For this review, take the finished solid that the model builds, in its own axes (mm). A direction names the side the tool comes from. Give positions to 0.01 mm unless a question says otherwise; leave off trailing zeros. Loops run counter-clockwise (first coordinate to the right, second up) from the corner with the lowest first, then second, coordinate; pieces in that order, holes last. Notation, with made-up numbers: (25, -29.5) - (60, -29.5) arc R18 cw to (60, -0.5) - close; hole circle Ø10 at (72, 72.5). An arc over 180 degrees is marked (long way). Answer in a Markdown table with one row per item.
Autodesk Inventor part; units mm, degrees
ref_plane "YZ Plane" through (0, 0, 0) normal (1, 0, 0) x (0, 1, 0)
ref_plane "XZ Plane" through (0, 0, 0) normal (0, 1, 0) x (-1, 0, 0)
ref_plane "XY Plane" through (0, 0, 0) normal (0, 0, 1) x (1, 0, 0)
sketch "Sketch3" plane through (0, 0, 0) normal (0, 0, 1) x (1, 0, 0)
  line L0 (225, 240) -> (-225, 240)
  line L1 (-225, 240) -> (-225, -240)
  line L2 (-225, -240) -> (225, -240)
  line L3 (225, -240) -> (225, 240)
  line L4 (225, 240) -> (-225, -240) construction
  line L5 (-225, 240) -> (225, -240) construction
  line L6 (150, 180) -> (-150, 180)
  line L7 (-150, 180) -> (-150, -180)
  line L8 (-150, -180) -> (150, -180)
  line L9 (150, -180) -> (150, 180)
  line L10 (150, 180) -> (-150, -180) construction
  line L11 (-150, 180) -> (150, -180) construction
  point P0 (0, 0)
  dimension "d22" = 450
  dimension "d23" = 480
  dimension "d24" = 300
  dimension "d25" = 360
extrude "Plate3" add sketch "Sketch3" along normal blind 10
sketch "Sketch4" plane through (0, 0, 0) normal (0, 0, -1) x (-1, 0, 0)
  circle A0 centre (0, 230) radius 6.5
  circle A1 centre (195, 230) radius 6.5
  circle A2 centre (-195, 230) radius 6.5
  circle A3 centre (-200, 160) radius 6.5
  circle A4 centre (-200, 0) radius 6
  circle A5 centre (-200, -160) radius 6
  circle A6 centre (-195, -230) radius 6
  circle A7 centre (0, -230) radius 6
  circle A8 centre (195, -230) radius 6
  circle A9 centre (200, -160) radius 6.5
  circle A10 centre (200, 0) radius 6.5
  circle A11 centre (200, 160) radius 6.5
  point P0 (0, 0)
extrude "Cut1" cut sketch "Sketch4" against normal blind 10
equation "\"d26\" = Thickness"
equation "\"d18\" = Thickness"
equation "\"BendReliefDepth\" = 0.5 * Thickness"
properties part number "NVPH-305 main flange"
1. For faces 4 (the face through (150, -3, 5)), 5 (the face through (3, 240, 5)), list the 3-axis set-ups (+Z, -Z, +X, -X, +Y, -Y) from which the entire face can be reached by the end or side of a thin tool; tool diameter is ignored.
Values:
| item | result |
|---|---|
| face 4 | +Z, -Z |
| face 5 | +Z, -Z, +X, -X, +Y |
2. We need section A-A, the plane y = 230. Give the boundary of the cut face in (x, z).
Values:
| item | result |
|---|---|
| outline | (-225, 0) - (-201.5, 0) - (-201.5, 10) - (-225, 10) - close; (-188.5, 0) - (-6.5, 0) - (-6.5, 10) - (-188.5, 10) - close; (6.5, 0) - (188.5, 0) - (188.5, 10) - (6.5, 10) - close; (201.5, 0) - (225, 0) - (225, 10) - (201.5, 10) - close |
3. Clearance check with a flat-ended pin moving along its axis: pin 1 (15 mm diameter, centred on x = 200, y = 160, fed in from -Z). State where the tip first meets the part, or that it passes through.
Values:
| item | result |
|---|---|
| pin 1 | stops at z = 0 |
4. Wall thickness on line 1 (Y direction, x = 132, z = 3); line 2 (X direction, y = -135, z = 2); line 3 (Y direction, x = -199.5, z = 2.75): over which ranges is each line inside the solid? List them lowest first. Write a range as [from, to].
Values:
| item | result |
|---|---|
| line 1 | y = [-240, -180], [180, 240] |
| line 2 | x = [-225, -150], [150, 225] |
| line 3 | y = [-240, -233.97], [-226.03, -166.48], [-153.52, -6.48], [6.48, 153.52], [166.48, 225.31], [234.69, 240] |
5. We need section D-D, the plane y = -84. Give the boundary of the cut face in (x, z), and give its area (3 significant figures).
Values:
| item | result |
|---|---|
| outline | (-225, 0) - (-150, 0) - (-150, 10) - (-225, 10) - close; (150, 0) - (225, 0) - (225, 10) - (150, 10) - close |
| area | 1,500 mm^2 |
6. Mouldability with a two-part tool opening along X and no side actions: class faces 1 (the face through (225, -3, 5)), 2 (the face through (-225, 3, 5)), 3 (the face through (-2, -180, 5)) as released by +X, released by -X, zero draft, split by the parting line, or undercut.
Values:
| item | result |
|---|---|
| face 1 | released by +X |
| face 2 | released by -X |
| face 3 | undercut |
7. We need section B-B, the plane x = 0. Give the boundary of the cut face in (y, z).
Values:
| item | result |
|---|---|
| outline | (-240, 0) - (-236, 0) - (-236, 10) - (-240, 10) - close; (-224, 0) - (-180, 0) - (-180, 10) - (-224, 10) - close; (180, 0) - (223.5, 0) - (223.5, 10) - (180, 10) - close; (236.5, 0) - (240, 0) - (240, 10) - (236.5, 10) - close |
8. We need section C-C, the plane z = 4.75. Count the separate pieces of the cut face and the enclosed holes in it, and give its area (3 significant figures).
Values:
| item | result |
|---|---|
| separate pieces | 1 |
| enclosed holes | 13 |
| area | 107,000 mm^2 |
